Input: part model. Units: mm. Frame: model coordinates. Round coordinates to 2 decimals unless told otherwise and drop trailing zeros. Loops run counter-clockwise (first coordinate to the right, second up) from the corner with the lowest first, then second, coordinate; pieces in that order, holes last.
(1) Cut plane C-C, the plane y = -12.5. Output: boundary loops of the cut face in (x, z).
(2) Cut plane A-A, the plane y = 0. Output: boundary loops of the cut face in (x, z).
(3) Line query: line 1 (Y direction, x = 0, z = 0.35); line 2 (Y direction, x = 0, z = 1.3); line 3 (Y direction, x = 10.5, z = 0.9). Output: solid intervals per line, ascending.
(4) Cut plane B-B, the plane y = -7. Give the number of separate pieces and of enclosed holes in the cut face, and give its area (3 significant figures).
(5) First-contact query: pin 1 Ø3 at (x, y) = (10.83, 6.25) entering from -Z. Flat tip, straight axial feed; report the tip coordinate or a pass-through.
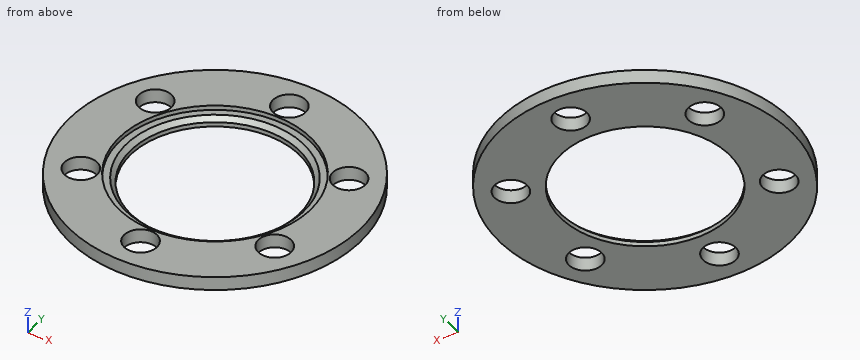
from build123d import *

# Parameters (mm, degrees)
F0_R     = 16
F0_R_2   = 1.8
F0_R_3   = 9.25
F1_DEPTH = 1.5
F2_R     = 10.5
F3_DEPTH = 0.5
F4_SIZE  = 0.5


with BuildPart() as f1:
    # F0 (on Top) → F1 (new body)
    with BuildSketch(Plane.XY):
        Circle(F0_R)
        with Locations((-10.825318, -6.25)):
            Circle(F0_R_2, mode=Mode.SUBTRACT)
        with Locations((0, -12.5)):
            Circle(F0_R_2, mode=Mode.SUBTRACT)
        with Locations((10.825318, -6.25)):
            Circle(F0_R_2, mode=Mode.SUBTRACT)
        with Locations((-10.825318, 6.25)):
            Circle(F0_R_2, mode=Mode.SUBTRACT)
        Circle(F0_R_3, mode=Mode.SUBTRACT)
        with Locations((10.825318, 6.25)):
            Circle(F0_R_2, mode=Mode.SUBTRACT)
        with Locations((0, 12.5)):
            Circle(F0_R_2, mode=Mode.SUBTRACT)
    extrude(amount=F1_DEPTH)

    # F2 (on face) → F3 (cut)
    with BuildSketch(Plane.XY.offset(1.5)):
        Circle(F2_R)
    extrude(amount=-F3_DEPTH, mode=Mode.SUBTRACT)

    # F4
    f4_edges = [f1.edges().sort_by_distance(p)[0] for p in [
        (-9.25, 0, 1),
    ]]
    chamfer(f4_edges, length=F4_SIZE)


solid = f1.part
Reported:
1. outline: (-9.99, 0) - (-1.8, 0) - (-1.8, 1.5) - (-9.99, 1.5) - close; (1.8, 0) - (9.99, 0) - (9.99, 1.5) - (1.8, 1.5) - close
2. outline: (-16, 0) - (-9.25, 0) - (-9.25, 0.5) - (-9.75, 1) - (-10.5, 1) - (-10.5, 1.5) - (-16, 1.5) - close; (9.25, 0) - (16, 0) - (16, 1.5) - (10.5, 1.5) - (10.5, 1) - (9.75, 1) - (9.25, 0.5) - close
3. line 1: y = -16 to -14.3, -10.7 to -9.25, 9.25 to 10.7, 14.3 to 16
3. line 2: y = -16 to -14.3, -10.7 to -10.5, 10.5 to 10.7, 14.3 to 16
3. line 3: y = -12.07 to -8.02, -4.48 to 4.48, 8.02 to 12.07
4. separate pieces: 4
4. enclosed holes: 0
4. area: 13.1 mm2
5. pin 1: passes through
